from build123d import *

# Parameters (mm, degrees)
ESQUISSE1_W             = 50
ESQUISSE1_H             = 80
BOSS_EXTRU_1_DEPTH      = 5
BOSS_EXTRU_2_START      = -42.4
ESQUISSE2_W             = 5
ESQUISSE2_H             = 12.2
ESQUISSE2_R             = 1.5
ESQUISSE2_W_2           = 5.01688185
BOSS_EXTRU_2_DEPTH      = 5
ESQUISSE3_R             = 3
ENL_V_MAT_EXTRU_1_DEPTH = 51.207967495
BOSS_EXTRU_3_START      = -10
ESQUISSE5_R             = 1.375
BOSS_EXTRU_3_DEPTH      = 5
ESQUISSE6_R             = 1.375
BOSS_EXTRU_4_DEPTH      = 10
BOSS_EXTRU_5_START      = -12.5
BOSS_EXTRU_5_DEPTH      = 10
CONG_1_R                = 5
CONG_2_R                = 5
CONG_3_R                = 5
CONG_1_OF_SYM_TRIE1_R   = 5
CONG_2_OF_SYM_TRIE1_R   = 5
CONG_3_OF_SYM_TRIE1_R   = 5
CHANFREIN1_SIZE         = 3
BOSS_EXTRU_6_DEPTH      = 5
ESQUISSE10_R            = 1.5
ENL_V_MAT_EXTRU_2_DEPTH = 64.767186518
CONG_4_R                = 10
CHANFREIN5_START        = -9.492908537
CHANFREIN5_OUTLINE_W    = 12
CHANFREIN5_OUTLINE_H    = 5
CHANFREIN5_DEPTH        = 4.242640687
CHANFREIN6_START        = 1.820799962
CHANFREIN6_OUTLINE_W    = 12
CHANFREIN6_OUTLINE_H    = 5
CHANFREIN6_DEPTH        = 4.242640687
CONG_5_START            = 25
CONG_5_DEPTH            = 5
CONG_6_START            = 25
CONG_6_DEPTH            = 5


with BuildPart() as part:
    # Esquisse1 → Boss.-Extru.1 (new body)
    with BuildSketch(Plane.XY):
        Rectangle(ESQUISSE1_W, ESQUISSE1_H)
    extrude(amount=BOSS_EXTRU_1_DEPTH)

    # Esquisse2 → Boss.-Extru.2 (add)
    # profile 1 of 2: a face of its own
    with BuildSketch(Plane(origin=(0, 40, 0), x_dir=(1, 0, 0), z_dir=(0, 1, 0)).offset(BOSS_EXTRU_2_START)):
        with Locations((17.5, 6.1)):
            Rectangle(ESQUISSE2_W, ESQUISSE2_H)
        with Locations(Location((17.5, 6.1, 0), (0, 0, 270))):
            Circle(ESQUISSE2_R, mode=Mode.SUBTRACT)
    # profile 2 of 2: a face of its own
    with BuildSketch(Plane(origin=(0, 40, 0), x_dir=(1, 0, 0), z_dir=(0, 1, 0)).offset(BOSS_EXTRU_2_START)):
        with Locations((-10.508440925, 6.1)):
            Rectangle(ESQUISSE2_W_2, ESQUISSE2_H)
        with Locations(Location((-10.5, 6.1, 0), (0, 0, 270))):
            Circle(ESQUISSE2_R, mode=Mode.SUBTRACT)
    extrude(amount=-BOSS_EXTRU_2_DEPTH)

    # Esquisse3 → Enlèv. mat.-Extru.1 (cut, through all)
    with BuildSketch(Plane.XY.offset(5)):
        Circle(ESQUISSE3_R)
    extrude(amount=-ENL_V_MAT_EXTRU_1_DEPTH, mode=Mode.SUBTRACT)

    # Esquisse5 → Boss.-Extru.3 (add)
    with BuildSketch(Plane(origin=(0, 40, 0), x_dir=(1, 0, 0), z_dir=(0, 1, 0)).offset(BOSS_EXTRU_3_START)):
        with BuildLine():
            Line((-7.425, 6.1), (-7.425, 0))
            Line((-7.425, 0), (2.575, 0))
            Line((2.575, 0), (2.575, 6.1))
            ThreePointArc((2.575, 6.1), (-2.425, 11.1), (-7.425, 6.1))
        make_face()
        with Locations(Location((-2.425, 6.1, 0), (0, 0, 270))):
            Circle(ESQUISSE5_R, mode=Mode.SUBTRACT)
    extrude(amount=-BOSS_EXTRU_3_DEPTH)

    # Esquisse6 → Boss.-Extru.4 (add)
    with BuildSketch(Plane(origin=(0, 30, 0), x_dir=(1, 0, 0), z_dir=(0, 1, 0))):
        with Locations(Location((-2.425, 6.1, 0), (0, 0, 270))):
            Circle(ESQUISSE6_R)
    extrude(amount=-BOSS_EXTRU_4_DEPTH)

    # Esquisse7 → Boss.-Extru.5 (add)
    with BuildSketch(Plane.XZ.offset(40).offset(BOSS_EXTRU_5_START)):
        with BuildLine():
            Line((10.577424804, 5), (10.577424804, 25.648245565))
            ThreePointArc((10.577424804, 25.648245565), (9.193748636, 28.673943766), (6, 29.606348721))
            Line((6, 29.606348721), (-5, 28.001622266))
            Line((-5, 28.001622266), (-5.721781005, 32.949251212))
            Line((-5.721781005, 32.949251212), (5.278218995, 34.553977666))
            ThreePointArc((5.278218995, 34.553977666), (12.464153425, 32.456066518), (15.577424804, 25.648245565))
            Line((15.577424804, 25.648245565), (15.577424804, 5))
            Line((15.577424804, 5), (10.577424804, 5))
        make_face()
    boss_extru_5 = extrude(amount=-BOSS_EXTRU_5_DEPTH)

    # Congé1
    cong_1_edges = [part.edges().sort_by_distance(p)[0] for p in [
        (15.577424804, -22.5, 5),
    ]]
    fillet(cong_1_edges, radius=CONG_1_R)

    # Congé2
    cong_2_edges = [part.edges().sort_by_distance(p)[0] for p in [
        (15.577424804, -17.5, 5),
    ]]
    fillet(cong_2_edges, radius=CONG_2_R)

    # Congé3
    cong_3_edges = [part.edges().sort_by_distance(p)[0] for p in [
        (15.577424804, -27.5, 5),
    ]]
    fillet(cong_3_edges, radius=CONG_3_R)

    # Symétrie1: Boss.-Extru.5 across plane
    add(boss_extru_5.mirror(Plane.ZX))

    # Congé1 of Symétrie1
    cong_1_of_sym_trie1_edges = [part.edges().sort_by_distance(p)[0] for p in [
        (15.577424804, 22.5, 5),
    ]]
    fillet(cong_1_of_sym_trie1_edges, radius=CONG_1_OF_SYM_TRIE1_R)

    # Congé2 of Symétrie1
    cong_2_of_sym_trie1_edges = [part.edges().sort_by_distance(p)[0] for p in [
        (15.577424804, 17.5, 5),
    ]]
    fillet(cong_2_of_sym_trie1_edges, radius=CONG_2_OF_SYM_TRIE1_R)

    # Congé3 of Symétrie1
    cong_3_of_sym_trie1_edges = [part.edges().sort_by_distance(p)[0] for p in [
        (15.577424804, 27.5, 5),
    ]]
    fillet(cong_3_of_sym_trie1_edges, radius=CONG_3_OF_SYM_TRIE1_R)

    # Chanfrein1
    chanfrein1_edges = [part.edges().sort_by_distance(p)[0] for p in [
        (-5.721781005, 22.5, 32.949251212),
        (-5.721781005, -22.5, 32.949251212),
    ]]
    chamfer(chanfrein1_edges, length=CHANFREIN1_SIZE)

    # Esquisse9 → Boss.-Extru.6 (add)
    with BuildSketch(Plane(origin=(0, -2.4, 0), x_dir=(1, 0, 0), z_dir=(0, 1, 0))):
        Polygon((-13.01688185, 12.2), (-25, 0), (-13.01688185, 0), align=None)
        Polygon((20, 12.2), (25, 0), (20, 0), align=None)
    extrude(amount=-BOSS_EXTRU_6_DEPTH)

    # Esquisse10 → Enlèv. mat.-Extru.2 (cut, through all)
    with BuildSketch(Plane.ZY.offset(-10.577424804)):
        with Locations((17.274122782, -22.5)):
            Circle(ESQUISSE10_R)
        with Locations((17.274122782, 22.5)):
            Circle(ESQUISSE10_R)
    extrude(amount=-ENL_V_MAT_EXTRU_2_DEPTH, mode=Mode.SUBTRACT)

    # Congé4
    cong_4_edges = [part.edges().sort_by_distance(p)[0] for p in [
        (25, -40, 2.5),
        (-25, -40, 2.5),
        (-25, 40, 2.5),
        (25, 40, 2.5),
    ]]
    fillet(cong_4_edges, radius=CONG_4_R)

    # Chanfrein5: read off the stored shape, not the designer's step
    # Chanfrein5 outline → Chanfrein5 (add)
    with BuildSketch(Plane(origin=(0, 0, 0), x_dir=(0.707106781186548, 0, -0.707106781186547), z_dir=(0.707106781186547, 0, 0.707106781186548)).offset(CHANFREIN5_START)):
        with Locations((-5, 27.5)):
            Rectangle(CHANFREIN5_OUTLINE_W, CHANFREIN5_OUTLINE_H)
    extrude(amount=CHANFREIN5_DEPTH)

    # Chanfrein6: read off the stored shape, not the designer's step
    # Chanfrein6 outline → Chanfrein6 (add)
    with BuildSketch(Plane(origin=(0, 0, 0), x_dir=(0.707106781186548, 0, 0.707106781186547), z_dir=(0.707106781186547, 0, -0.707106781186548)).offset(CHANFREIN6_START)):
        with Locations((2, -27.5)):
            Rectangle(CHANFREIN6_OUTLINE_W, CHANFREIN6_OUTLINE_H)
    extrude(amount=CHANFREIN6_DEPTH)

    # Congé5: read off the stored shape, not the designer's step
    # Congé5 outline → Congé5 (add)
    with BuildSketch(Plane(origin=(0, 0, 0), x_dir=(1, 0, 0), z_dir=(0, 1, 0)).offset(CONG_5_START)):
        with BuildLine():
            ThreePointArc((-6.755521581, 8.599316474), (-9.663638899, 4.245895741), (-13.11542298, 0.30957702))
            Line((-13.11542298, 0.30957702), (-7.425, 6))
            Line((-7.425, 6), (-7.425, 6.1))
            ThreePointArc((-7.425, 6.1), (-7.254731251, 7.393714052), (-6.755521581, 8.599316474))
        make_face()
    extrude(amount=CONG_5_DEPTH)

    # Congé6: read off the stored shape, not the designer's step
    # Congé6 outline → Congé6 (add)
    with BuildSketch(Plane(origin=(0, 0, 0), x_dir=(1, 0, 0), z_dir=(0, 1, 0)).offset(CONG_6_START)):
        with BuildLine():
            ThreePointArc((8.26542298, 0.30957702), (4.813638899, 4.245895741), (1.905521581, 8.599316474))
            ThreePointArc((1.905521581, 8.599316474), (2.40473125, 7.393714052), (2.575, 6.1))
            Line((2.575, 6.1), (2.575, 6))
            Line((2.575, 6), (8.26542298, 0.30957702))
        make_face()
    extrude(amount=CONG_6_DEPTH)


solid = part.part
Could you check a few things on this model? Use its own coordinates, in mm. A direction names the side the tool comes from. Coordinates: 2 decimals unless noted, no trailing zeros. Order: outer loops, then holes, each group sorted by start corner. A loop starts at its lowest first (then second) coordinate and runs counter-clockwise, first axis right, second up.
Q1. Will these pins go through, and if not, where does the flat tip stop? pin 1 (12 mm diameter, centred on x = 2.5, z = 28, fed in from -Y); pin 2 (3 mm diameter, centred on y = 21.5, z = 14.5, fed in from +X); pin 3 (5.5 mm diameter, centred on x = -0.5, z = -5, fed in from -Y).
Q2. Please list where these lines run through material, in increasing order: L1, parallel to Y at x = 0, z = 1.2; L2, parallel to Z at x = 6.5, y = -23.5; L3, parallel to X at y = -5.6, z = -6.1.
Q3. Suppose I cut it at D-D on x = 17.5. Please give me the cut outline in (y, z).
Q4. Suppose I cut it at C-C on z = 4. Please give me the cut outline in (x, y).
Q5. Suppose I cut it at A-A on z = 22. Please give me the cut outline in (x, y).
Q6. Thinking about a two-plate mould opening in Z: for faces 4 (the cylindrical face through (-22.15, 36.99, 2.54)), 5 (the cylindrical face through (12.38, 22.57, 32.53)), 6 (the flat face through (10.577, -23, 15)), which applies, released by +Z, released by -Z, zero draft, split by the parting line, or undercut?
Q7. Suppose I cut it at B-B on y = -22.5. Please give me the cut outline in (x, z).
Q8. Which directions (+Z, -Z, +X, -X, +Y, -Y) give clear straight access to the entire face, cutting with the end or side of a thin tool? Please do faces 1 (the cylindrical face through (-3.26, 22.54, -7.19)), 2 (the flat face through (15.577, 23, 20)), 3 (the flat face through (-2, 20, -6)).
Answer:
1. pin 1: stops at y = -27.5
1. pin 2: stops at x = 15.58
1. pin 3: stops at y = 20
2. L1: y = -40 to -3, 3 to 40
2. L2: z = 0 to 5, 29.65 to 34.65
2. L3: x = -19.01 to -12, -9 to -8, 15 to 16, 19 to 22.5
3. outline: (-39.68, 0) - (-7.4, 0) - (-7.4, -4.6) - (-2.4, -4.6) - (-2.4, 0) - (39.68, 0) - (39.68, 5) - (32.5, 5) arc R5 cw to (29.42, 6.06) - (15.58, 6.06) arc R5 cw to (12.5, 5) - (-12.5, 5) arc R5 cw to (-15.58, 6.06) - (-29.42, 6.06) arc R5 cw to (-32.5, 5) - (-39.68, 5) - close; (-7.4, -12.2) - (-2.4, -12.2) - (-2.4, -7.6) - (-7.4, -7.6) - close
4. outline: (-25, -30) arc R10 ccw to (-15, -40) - (15, -40) arc R10 ccw to (25, -30) - (25, 30) arc R10 ccw to (15, 40) - (-15, 40) arc R10 ccw to (-25, 30) - close; hole circle Ø6 at (0, 0)
5. outline: (10.58, -27.5) - (15.58, -27.5) - (15.58, -17.5) - (10.58, -17.5) - close; (10.58, 17.5) - (15.58, 17.5) - (15.58, 27.5) - (10.58, 27.5) - close
6. face 4: zero draft
6. face 5: released by +Z
6. face 6: undercut
7. outline: (-25, 0) - (25, 0) - (25, 5) - (20.58, 5) arc R5 cw to (15.58, 10) - (15.58, 15.77) - (10.58, 15.77) - (10.58, 5) - (-25, 5) - close; (-5.29, 29.98) - (-5, 28) - (6, 29.61) arc R4 cw to (10.58, 25.65) - (10.58, 18.77) - (15.58, 18.77) - (15.58, 25.65) arc R9 ccw to (5.28, 34.55) - (-2.75, 33.38) - close
8. face 1: -Y
8. face 2: +Z, +X, +Y, -Y
8. face 3: -Z, +X, -X, -Y
